Input: part model. Units: mm. Frame: model coordinates. Give positions to 0.01 mm unless a question says otherwise; leave off trailing zeros. Loops run counter-clockwise (first coordinate to the right, second up) from the corner with the lowest first, then second, coordinate; pieces in that order, holes last. Notation, with made-up numbers: (-8.75, 17) - (21.25, 17) arc R15 ccw to (21.25, 30) - close; hole circle Ø10 at (48, -3.5). An arc over 180 degrees is marked (long way). One line per item, written item: value.
Autodesk Inventor part; units mm, degrees
ref_plane "YZ Plane" through (0, 0, 0) normal (1, 0, 0) x (0, 1, 0)
ref_plane "XZ Plane" through (0, 0, 0) normal (0, 1, 0) x (-1, 0, 0)
ref_plane "XY Plane" through (0, 0, 0) normal (0, 0, 1) x (1, 0, 0)
sketch "Sketch1" plane through (0, 0, 0) normal (0, 1, 0) x (-1, 0, 0)
  circle A0 centre (0, 0) radius 13
  line L0 (28.6148, 9.0106) -> (-45.3852, 244.0106)
  line L1 (-104, 235) -> (-104, 75.4136)
  circle A1 centre (-74, 235) radius 12.5
  circle A2 centre (-74, 0) radius 12.5 construction
  line L2 (0, 0) -> (-74, 0)
  line L3 (28.6148, -9.0106) -> (-45.3852, -244.0106)
  line L4 (-104, -235) -> (-104, 75.4136)
  circle A3 centre (-74, -235) radius 12.5
  arc A4 (-45.3852, 244.0106) -> (-104, 235) centre (-74, 235) ccw
  arc A5 (28.6148, -9.0106) -> (28.6148, 9.0106) centre (0, 0) ccw
  arc A6 (-104, -235) -> (-45.3852, -244.0106) centre (-74, -235) ccw
  point P0 (-104, 430.1523)
  point P1 (-104, -430.1523)
  dimension "d0" = 26
  dimension "d1" = 25
  dimension "d2" = 25
  dimension "d4" = 74
  dimension "d6" = 470
  dimension "d9" = 30
  dimension "d10" = 30
extrude "Extrusion1" add sketch "Sketch1" along normal mid plane 25.4
properties part number "Espacador_Delta"
Item 1: Section B-B, the plane y = 8.5. Output: boundary loops of the cut face in (x, z), and give its area (3 significant figures).
Verdict:
outline: (-28.61, -9.01) - (45.39, -244.01) arc R30 ccw to (104, -235) - (104, 235) arc R30 ccw to (45.39, 244.01) - (-28.61, 9.01) arc R30 ccw to start; hole circle Ø26 at (0, 0); hole circle Ø25 at (74, -235); hole circle Ø25 at (74, 235)
area: 47,600 mm^2
Item 2: Draft query along X for faces 1 (the face through (7.87, -0.18, -124.87)), 2 (the face through (53, -12.7, 4)), 3 (the face through (75.627, -0.178, -247.394)). Return one class per face: pulls with the +X half, pulls with the -X half, needs draft (parallel to the pull), parting line crosses it, or undercut.
Verdict:
face 1: pulls with the -X half
face 2: needs draft
face 3: undercut
Item 3: Section D-D, the plane x = 3. Output: boundary loops of the cut face in (y, z), and give its area (3 significant figures).
Verdict:
outline: (-12.7, -109.41) - (12.7, -109.41) - (12.7, -12.65) - (-12.7, -12.65) - close; (-12.7, 12.65) - (12.7, 12.65) - (12.7, 109.41) - (-12.7, 109.41) - close
area: 4,920 mm^2
Item 4: Section C-C, the plane z = 0. Output: boundary loops of the cut face in (x, y).
Verdict:
outline: (-30, -12.7) - (-13, -12.7) - (-13, 12.7) - (-30, 12.7) - close; (13, -12.7) - (104, -12.7) - (104, 12.7) - (13, 12.7) - close
Item 5: Material intervals for L1, parallel to Z at x = 74, y = 0.25; L2, parallel to Z at x = 80.5, y = 9.25; L3, parallel to X at y = -3.5, z = -225.5, sorted ascending.
Verdict:
L1: z = -265 to -247.5, -222.5 to 222.5, 247.5 to 265
L2: z = -264.29 to -245.68, -224.32 to 224.32, 245.68 to 264.29
L3: x = 39.56 to 65.88, 82.12 to 104
Item 6: Section A-A, the plane x = 74. Output: boundary loops of the cut face in (y, z).
Verdict:
outline: (-12.7, -265) - (12.7, -265) - (12.7, -247.5) - (-12.7, -247.5) - close; (-12.7, -222.5) - (12.7, -222.5) - (12.7, 222.5) - (-12.7, 222.5) - close; (-12.7, 247.5) - (12.7, 247.5) - (12.7, 265) - (-12.7, 265) - close
Item 7: Pin query (flat end, axial travel): P1, Ø4, axis at x = 64.5, y = 9, coming from the +Z side; P2, Ø3, axis at y = -2, z = -201.5, coming from the -X side; P3, Ø5, axis at y = 6.5, z = 133.5, coming from the -X side. Return the tip coordinate at first contact, or that it passes through.
Verdict:
P1: stops at z = 264.05
P2: stops at x = 31.53
P3: stops at x = 9.8
